```python
from build123d import *

# Parameters (mm, degrees)
SKETCH_W        = 78
SKETCH_H        = 95
PAD_DEPTH       = 1.5
SKETCH002_W     = 14
SKETCH002_H     = 14
POCKET_DEPTH    = 1.501
FILLET_R        = 1
SKETCH003_R     = 3
POCKET001_DEPTH = 1.501
FILLET001_R     = 5


with BuildPart() as part:
    # Sketch → Pad (new body)
    with BuildSketch(Plane.XY):
        Rectangle(SKETCH_W, SKETCH_H)
    extrude(amount=PAD_DEPTH)

    # Sketch002 (on Face6 of Pad) → Pocket (cut, through all)
    with BuildSketch(Plane.XY.offset(1.5)):
        with Locations((-20, 20)):
            Rectangle(SKETCH002_W, SKETCH002_H)
        with Locations((0, 20)):
            Rectangle(SKETCH002_W, SKETCH002_H)
        with Locations((20, 20)):
            Rectangle(SKETCH002_W, SKETCH002_H)
        with Locations((-20, 0)):
            Rectangle(SKETCH002_W, SKETCH002_H)
        Rectangle(SKETCH002_W, SKETCH002_H)
        with Locations((20, 0)):
            Rectangle(SKETCH002_W, SKETCH002_H)
        with Locations((-20, -20)):
            Rectangle(SKETCH002_W, SKETCH002_H)
        with Locations((0, -20)):
            Rectangle(SKETCH002_W, SKETCH002_H)
        with Locations((20, -20)):
            Rectangle(SKETCH002_W, SKETCH002_H)
    extrude(amount=-POCKET_DEPTH, mode=Mode.SUBTRACT)

    # Fillet
    fillet_edges = [part.edges().sort_by_distance(p)[0] for p in [
        (-27, 27, 0.75),
        (-27, 7, 0.75),
        (-27, -13, 0.75),
        (-7, 27, 0.75),
        (-7, 7, 0.75),
        (-7, -13, 0.75),
        (13, -13, 0.75),
        (13, 7, 0.75),
        (13, 27, 0.75),
        (-13, 27, 0.75),
        (7, 27, 0.75),
        (27, 27, 0.75),
        (-13, 7, 0.75),
        (7, 7, 0.75),
        (27, 7, 0.75),
        (-13, -13, 0.75),
        (7, -13, 0.75),
        (27, -13, 0.75),
        (27, 13, 0.75),
        (7, 13, 0.75),
        (-13, 13, 0.75),
        (27, -7, 0.75),
        (7, -7, 0.75),
        (-13, -7, 0.75),
        (27, -27, 0.75),
        (7, -27, 0.75),
        (-13, -27, 0.75),
        (13, -27, 0.75),
        (-7, -27, 0.75),
        (-27, -27, 0.75),
        (13, -7, 0.75),
        (-7, -7, 0.75),
        (-27, -7, 0.75),
        (13, 13, 0.75),
        (-7, 13, 0.75),
        (-27, 13, 0.75),
    ]]
    fillet(fillet_edges, radius=FILLET_R)

    # Sketch003 (on Face78 of Fillet) → Pocket001 (cut, through all)
    with BuildSketch(Plane.XY.offset(1.5)):
        with Locations((-31, 39.5)):
            Circle(SKETCH003_R)
        with Locations((31, 39.5)):
            Circle(SKETCH003_R)
        with Locations((31, -39.5)):
            Circle(SKETCH003_R)
        with Locations((-31, -39.5)):
            Circle(SKETCH003_R)
    extrude(amount=-POCKET001_DEPTH, mode=Mode.SUBTRACT)

    # Fillet001
    fillet001_edges = [part.edges().sort_by_distance(p)[0] for p in [
        (39, -47.5, 0.75),
        (-39, -47.5, 0.75),
        (-39, 47.5, 0.75),
        (39, 47.5, 0.75),
    ]]
    fillet(fillet001_edges, radius=FILLET001_R)


solid = part.part
```
For this review, take the finished solid that the model builds, in its own axes (mm). Round coordinates to 2 decimals unless told otherwise and drop trailing zeros. Write each loop counter-clockwise with the first axis right and the second up, starting at its lowest first coordinate (ties: lowest second). Pieces come first, ordered by that corner, then holes.
1) Mouldability with a two-part tool opening along Y and no side actions: class faces 1 (the face through (28.79, -37.47, 0.76)), 2 (the face through (-37.57, 46, 0.76)), 3 (the face through (37.5, -46.07, 0.76)), 4 (the face through (-9, 1, 1.5)) as +Y half, -Y half, draft (parallel to the pull), parting line (faces both ways), or undercut.
Answer below:
face 1: undercut
face 2: +Y half
face 3: -Y half
face 4: draft
2) For line 1 along Y through (x, z) = (-3.5, 1.15); line 2 along Y through (x, z) = (-31, 0.3); line 3 along X through (y, z) = (6, 0.75), list the stretches that pass through material, from the lowest coordinate up.
Answer below:
line 1: y = -47.5 to -27, -13 to -7, 7 to 13, 27 to 47.5
line 2: y = -47.5 to -42.5, -36.5 to 36.5, 42.5 to 47.5
line 3: x = -39 to -27, -13 to -7, 7 to 13, 27 to 39
3) Take a section at A-A on x = 1. Give the boundary of the cut face in (y, z), then the cut area to 3 significant figures.
Answer below:
outline: (-47.5, 0) - (-27, 0) - (-27, 1.5) - (-47.5, 1.5) - close; (-13, 0) - (-7, 0) - (-7, 1.5) - (-13, 1.5) - close; (7, 0) - (13, 0) - (13, 1.5) - (7, 1.5) - close; (27, 0) - (47.5, 0) - (47.5, 1.5) - (27, 1.5) - close
area: 79.5 mm2
4) Take a section at C-C on x = 31. Give the boundary of the cut face in (y, z), then the cut area to 4 significant figures.
Answer below:
outline: (-47.5, 0) - (-42.5, 0) - (-42.5, 1.5) - (-47.5, 1.5) - close; (-36.5, 0) - (36.5, 0) - (36.5, 1.5) - (-36.5, 1.5) - close; (42.5, 0) - (47.5, 0) - (47.5, 1.5) - (42.5, 1.5) - close
area: 124.5 mm2
5) Take a section at D-D on y = 3. Give the boundary of the cut face in (x, z).
Answer below:
outline: (-39, 0) - (-27, 0) - (-27, 1.5) - (-39, 1.5) - close; (-13, 0) - (-7, 0) - (-7, 1.5) - (-13, 1.5) - close; (7, 0) - (13, 0) - (13, 1.5) - (7, 1.5) - close; (27, 0) - (39, 0) - (39, 1.5) - (27, 1.5) - close
6) Take a section at B-B on y = -39.5. Give the boundary of the cut face in (x, z).
Answer below:
outline: (-39, 0) - (-34, 0) - (-34, 1.5) - (-39, 1.5) - close; (-28, 0) - (28, 0) - (28, 1.5) - (-28, 1.5) - close; (34, 0) - (39, 0) - (39, 1.5) - (34, 1.5) - close
